from build123d import *

# Parameters (mm, degrees)
F0_W     = 76.2
F0_H     = 101.6
F1_DEPTH = 254
F3_DEPTH = 254
F4_T     = -5.08
F5_W     = 47.115137
F5_H     = 73.164374
F6_DEPTH = 5.08


with BuildPart() as f1:
    # F0 (on Front) → F1 (new body)
    with BuildSketch(Plane.XZ):
        with Locations((-38.1, 50.8)):
            Rectangle(F0_W, F0_H)
    extrude(amount=F1_DEPTH)

    # F2 (on face) → F3 (join)
    with BuildSketch(Plane.XZ.offset(254)):
        Polygon((-40.087454, 135.909051), (-76.2, 101.6), (0, 101.6), align=None)
    extrude(amount=-F3_DEPTH)

    # F4
    f4_openings = [f1.faces().sort_by_distance(p)[0] for p in [
        (-38.1, -127, 0),
    ]]
    offset(amount=F4_T, openings=f4_openings)

    # F5 (on face) → F6 (cut, through all)
    with BuildSketch(Plane.XZ.offset(254)):
        with Locations((-38.100001, 36.582187)):
            Rectangle(F5_W, F5_H)
    extrude(amount=-F6_DEPTH, mode=Mode.SUBTRACT)


solid = f1.part
Could you check a few things on this model? Use its own coordinates, in mm. A direction names the side the tool comes from. Round coordinates to 2 decimals unless told otherwise and drop trailing zeros. Write each loop counter-clockwise with the first axis right and the second up, starting at its lowest first coordinate (ties: lowest second). Pieces come first, ordered by that corner, then holes. Notation, with made-up numbers: (37.25, 38) - (77.25, 38) arc R23 cw to (77.25, 47) - close; hole circle Ø1 at (18, 43.25). An arc over 180 degrees is marked (long way). Use a Markdown table: item, result.
Q1. Please list where these lines run through material, in increasing order: L1, parallel to X at y = -19, z = 51; L2, parallel to Y at x = -34, z = 74.5; L3, parallel to X at y = -146.5, z = 101.5.
Output values:
| item | result |
|---|---|
| L1 | -76.2 to -71.12, -5.08 to 0 |
| L2 | -254 to -248.92, -5.08 to 0 |
| L3 | -76.2 to -68.93, -7.7 to 0 |
Q2. Thinking about a two-plate mould opening in X: for faces 1 (the flat face through (-57.891, -128.778, 118.995)), 2 (the flat face through (-39, -254, 84)), 3 (the flat face through (-39, -248.92, 80)), which applies, released by +X, released by -X, zero draft, split by the parting line, or undercut?
Output values:
| item | result |
|---|---|
| face 1 | released by -X |
| face 2 | zero draft |
| face 3 | undercut |
Q3. I want a section at D-D (z = 41). List the corners of the cut face in (x, y) for me, plus the area to 3 significant figures.
Output values:
| item | result |
|---|---|
| outline | (-76.2, -254) - (-61.66, -254) - (-61.66, -248.92) - (-71.12, -248.92) - (-71.12, -5.08) - (-5.08, -5.08) - (-5.08, -248.92) - (-14.54, -248.92) - (-14.54, -254) - (0, -254) - (0, 0) - (-76.2, 0) - close |
| area | 3,010 mm2 |
Q4. For faces 4 (the flat face through (-38, -251, 73.164)), 5 (the flat face through (-39, 0, 54)), 6 (the flat face through (-5.08, -125, 49)), which set-ups out of +Z, -Z, +X, -X, +Y, -Y let a thin tool reach every point of the face, with its end or its side?
Output values:
| item | result |
|---|---|
| face 4 | -Z, -Y |
| face 5 | +Z, -Z, +X, -X, +Y |
| face 6 | -Z |
Q5. I want a section at A-A (z = 80). List the corners of the cut face in (x, y) for me.
Output values:
| item | result |
|---|---|
| outline | (-76.2, -254) - (0, -254) - (0, 0) - (-76.2, 0) - close; hole (-71.12, -248.92) - (-5.08, -248.92) - (-5.08, -5.08) - (-71.12, -5.08) - close |
Q6. For pin 1 (5 mm diameter, centred on y = -51.5, z = 114.5, fed in from +X); pin 2 (10 mm diameter, centred on x = -39, y = -65, fed in from -Z); pin 3 (5 mm diameter, centred on x = -29.5, z = 37, fed in from +Y); pin 4 (5 mm diameter, centred on x = -13, y = -201.5, fed in from -Z), each with a flat end and sliding along its axis, tell me the tip position at first contact or that it passes through.
Output values:
| item | result |
|---|---|
| pin 1 | x = -12.15 |
| pin 2 | z = 124.01 |
| pin 3 | y = 0 |
| pin 4 | z = 103.9 |
Q7. I want a section at C-C (x = -27.5). List the corners of the cut face in (y, z) for me, plus the area to 3 significant figures.
Output values:
| item | result |
|---|---|
| outline | (-254, 73.16) - (-248.92, 73.16) - (-248.92, 118.45) - (-5.08, 118.45) - (-5.08, 0) - (0, 0) - (0, 125.14) - (-254, 125.14) - close |
| area | 2,530 mm2 |
Q8. I want a section at B-B (y = -184.5). List the corners of the cut face in (x, z) for me, plus the area to 3 significant figures.
Output values:
| item | result |
|---|---|
| outline | (-76.2, 0) - (-71.12, 0) - (-71.12, 99.42) - (-39.91, 129.07) - (-5.08, 99.26) - (-5.08, 0) - (0, 0) - (0, 101.6) - (-40.09, 135.91) - (-76.2, 101.6) - close |
| area | 1,510 mm2 |
